Input: part model. Units: mm. Frame: model coordinates. Face numbers are marked on the shaded views. A direction names the side the tool comes from. Coordinates: 2 decimals unless noted, no trailing zeros. Order: outer loops, then holes, each group sorted by start corner. A loop starts at its lowest first (then second) coordinate and runs counter-clockwise, first axis right, second up. Notation, with made-up numbers: (-32, 50.25) -> (23, 50.25) arc R17 ccw to (23, 57.25) -> close; hole circle Ø1 at (-5.75, 36). An arc over 180 degrees is marked (long way). One line per item, written item: value. Start each with the question number.
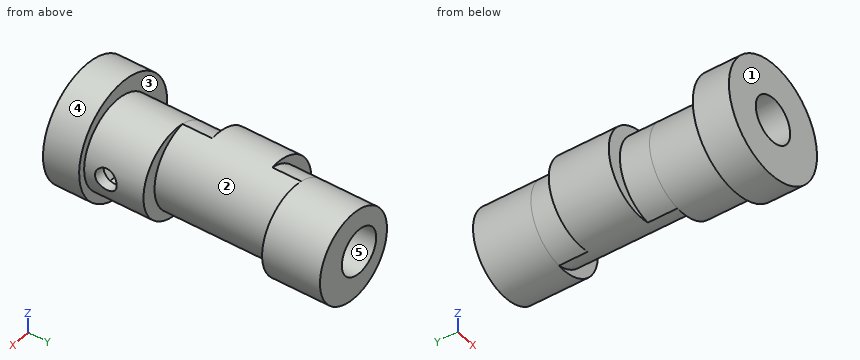
from build123d import *

# Parameters (mm, degrees)
SKETCH1_R           = 7.95
BOSS_EXTRUDE1_DEPTH = 5
SKETCH2_R           = 6.05
BOSS_EXTRUDE2_DEPTH = 8.2
SKETCH3_R           = 6.05
BOSS_EXTRUDE3_DEPTH = 16.4
CUT_EXTRUDE1_DEPTH  = 4.1
SKETCH5_R           = 6.05
BOSS_EXTRUDE4_DEPTH = 8
CUT_EXTRUDE2_START  = -4
CUT_EXTRUDE2_DEPTH  = 4
SKETCH7_R           = 3.1
CUT_EXTRUDE3_DEPTH  = 40.244935979
SKETCH8_R           = 1.5
CUT_EXTRUDE4_DEPTH  = 40.244935979
SKETCH9_R           = 1.5
CUT_EXTRUDE5_DEPTH  = 5.5


with BuildPart() as part:
    # Sketch1 → Boss-Extrude1 (new body)
    with BuildSketch(Plane(origin=(0, 0, 0), x_dir=(1, 0, 0), z_dir=(0, 1, 0))):
        with Locations(Location((0, 0, 0), (0, 0, 270))):
            Circle(SKETCH1_R)
    extrude(amount=BOSS_EXTRUDE1_DEPTH)

    # Sketch2 → Boss-Extrude2 (add)
    with BuildSketch(Plane(origin=(0, 5, 0), x_dir=(1, 0, 0), z_dir=(0, 1, 0))):
        with Locations(Location((1, 0, 0), (0, 0, 270))):
            Circle(SKETCH2_R)
    extrude(amount=BOSS_EXTRUDE2_DEPTH)

    # Sketch3 → Boss-Extrude3 (add)
    with BuildSketch(Plane(origin=(0, 13.2, 0), x_dir=(1, 0, 0), z_dir=(0, 1, 0))):
        with Locations(Location((-1, 0, 0), (0, 0, 80.485961644))):
            Circle(SKETCH3_R)
    extrude(amount=BOSS_EXTRUDE3_DEPTH)

    # Sketch4 → Cut-Extrude1 (cut)
    with BuildSketch(Plane.XZ.offset(-13.2)):
        with BuildLine():
            ThreePointArc((0, 5.966783053), (-7.05, 0), (0, -5.966783053))
            ThreePointArc((0, -5.966783053), (-5.05, 0), (0, 5.966783053))
        make_face()
    extrude(amount=-CUT_EXTRUDE1_DEPTH, mode=Mode.SUBTRACT)

    # Sketch5 → Boss-Extrude4 (add)
    with BuildSketch(Plane(origin=(0, 29.6, 0), x_dir=(1, 0, 0), z_dir=(0, 1, 0))):
        with Locations(Location((1, 0, 0), (0, 0, 99.514038356))):
            Circle(SKETCH5_R)
    extrude(amount=BOSS_EXTRUDE4_DEPTH)

    # Sketch6 → Cut-Extrude2 (cut)
    with BuildSketch(Plane(origin=(0, 29.6, 0), x_dir=(1, 0, 0), z_dir=(0, 1, 0)).offset(CUT_EXTRUDE2_START)):
        with BuildLine():
            ThreePointArc((0, 5.966783053), (-5.05, 0), (0, -5.966783053))
            ThreePointArc((0, -5.966783053), (-7.05, 0), (0, 5.966783053))
        make_face()
    extrude(amount=CUT_EXTRUDE2_DEPTH, mode=Mode.SUBTRACT)

    # Sketch7 → Cut-Extrude3 (cut, through all)
    with BuildSketch(Plane.XZ):
        with Locations(Location((0, 0, 0), (0, 0, 270))):
            Circle(SKETCH7_R)
    extrude(amount=-CUT_EXTRUDE3_DEPTH, mode=Mode.SUBTRACT)

    # Sketch8 → Cut-Extrude4 (cut, through all)
    with BuildSketch(Plane(origin=(0, 0, 0), x_dir=(0, 0, -1), z_dir=(1, 0, 0))):
        with Locations(Location((0, 8, 0), (0, 0, 180))):
            Circle(SKETCH8_R)
    extrude(amount=CUT_EXTRUDE4_DEPTH, mode=Mode.SUBTRACT)

    # Sketch9 → Cut-Extrude5 (cut)
    with BuildSketch(Plane(origin=(0, 0, 0), x_dir=(0, 0, -1), z_dir=(1, 0, 0))):
        Polygon((0, 11.175426481), (-2.75, 9.58771324), (-2.75, 6.41228676), (0, 4.824573519), (2.75, 6.41228676), (2.75, 9.58771324), align=None)
        with Locations(Location((0, 8, 0), (0, 0, 180))):
            Circle(SKETCH9_R, mode=Mode.SUBTRACT)
    extrude(amount=CUT_EXTRUDE5_DEPTH, mode=Mode.SUBTRACT)


solid = part.part
1) Pin query (flat end, axial travel): pin 1 Ø3.5 at (y, z) = (8, 0) entering from -X; pin 2 Ø6 at (y, z) = (29.5, 1) entering from +X; pin 3 Ø1.5 at (y, z) = (20.5, 3.5) entering from +X. Return the tip coordinate at first contact, or that it passes through.
2) Section query B-B, the plane z = -2.25. Return the cut outline in (x, y), plus the area to 3 significant figures.
3) Section query C-C, the plane y = 10.5. Return the cut outline in (x, z), plus the area to 3 significant figures.
4) Section query D-D, the plane z = 4.5. Return the cut outline in (x, y), plus the area to 3 significant figures.
5) Section query A-A, the plane x = -0.5. Return the cut outline in (y, z).
6) Access query for the marked faces 1 and 2. Directions: +Z, -Z, +X, -X, +Y, -Y. A direction counts if a zero-diameter tool reaches every point of the face in a straight line with its end or side. Return the directions, or none.
7) Mould query, pull axis Z, two halves, no side actions, for the marked faces 3, 4 and 5. Classes: +Z half, -Z half, draft (parallel to the pull), parting line (faces both ways), or undercut.
8) Ray query, line 1 along Y through (x, z) = (6.75, 0); line 2 along Y through (x, z) = (3, 5.5); line 3 along X through (y, z) = (23, 0). Return the intervals inside material, ascending. Write a range as from..to.
Entries:
1. pin 1: stops at x = -5.05
1. pin 2: stops at x = 7.05
1. pin 3: stops at x = 4.39
2. outline: (-7.62, 0) -> (-2.13, 0) -> (-2.13, 37.6) -> (-4.62, 37.6) -> (-4.62, 25.6) -> (-6.62, 25.6) -> (-6.62, 17.3) -> (-4.62, 17.3) -> (-4.62, 5) -> (-7.62, 5) -> close; (2.13, 0) -> (7.62, 0) -> (7.62, 5) -> (6.62, 5) -> (6.62, 13.2) -> (4.62, 13.2) -> (4.62, 29.6) -> (6.62, 29.6) -> (6.62, 37.6) -> (2.13, 37.6) -> (2.13, 9.88) -> (5.5, 9.88) -> (5.5, 6.12) -> (2.13, 6.12) -> close
2. area: 253 mm2
3. outline: circle Ø12.1 at (1, 0); hole (2.87, -1.17) -> (5.5, -1.17) -> (5.5, 1.17) -> (2.87, 1.17) arc R3.1 ccw (long way) to start
3. area: 79.0 mm2
4. outline: (-6.55, 0) -> (6.55, 0) -> (6.55, 5) -> (5.04, 5) -> (5.04, 13.2) -> (3.04, 13.2) -> (3.04, 29.6) -> (5.04, 29.6) -> (5.04, 37.6) -> (-3.04, 37.6) -> (-3.04, 25.6) -> (-5.04, 25.6) -> (-5.04, 17.3) -> (-3.04, 17.3) -> (-3.04, 5) -> (-6.55, 5) -> close
4. area: 313 mm2
5. outline: (0, -7.93) -> (5, -7.93) -> (5, -5.86) -> (17.3, -5.86) -> (17.3, -6.03) -> (25.6, -6.03) -> (25.6, -5.86) -> (37.6, -5.86) -> (37.6, -3.06) -> (0, -3.06) -> close; (0, 3.06) -> (37.6, 3.06) -> (37.6, 5.86) -> (25.6, 5.86) -> (25.6, 6.03) -> (17.3, 6.03) -> (17.3, 5.86) -> (5, 5.86) -> (5, 7.93) -> (0, 7.93) -> close
6. face 1: +Z, -Z, +X, -X, -Y
6. face 2: none
7. face 3: draft
7. face 4: parting line
7. face 5: undercut
8. line 1: y = 0..6.5, 9.5..13.2, 29.6..37.6
8. line 2: y = 0..13.2, 29.6..37.6
8. line 3: x = -7.05..-3.1, 3.1..5.05
